from build123d import *

# Parameters (mm, degrees)
SKETCH2_R           = 2.5
BOSS_EXTRUDE1_DEPTH = 3.8
SKETCH3_R           = 2.95
BOSS_EXTRUDE3_DEPTH = 1
SKETCH4_W           = 0.865778577
SKETCH4_H           = 6.939291368
CUT_EXTRUDE1_DEPTH  = 1


with BuildPart() as part:
    # Sketch2 → Boss-Extrude1 (new, symmetric)
    with BuildSketch(Plane(origin=(0, 0, 0), x_dir=(0, 0, -1), z_dir=(1, 0, 0))):
        with Locations(Location((0, 0, 0), (0, 0, 180))):
            Circle(SKETCH2_R)
    extrude(amount=BOSS_EXTRUDE1_DEPTH, both=True)

    # Sketch3 → Boss-Extrude3 (add)
    with BuildSketch(Plane(origin=(3.8, 0, 0), x_dir=(0, 0, -1), z_dir=(1, 0, 0))):
        Circle(SKETCH3_R)
    extrude(amount=BOSS_EXTRUDE3_DEPTH)

    # Sketch4 → Cut-Extrude1 (cut)
    with BuildSketch(Plane.ZY.offset(-3.8)):
        with Locations((-2.932889289, -0.568577956)):
            Rectangle(SKETCH4_W, SKETCH4_H)
    extrude(amount=-CUT_EXTRUDE1_DEPTH, mode=Mode.SUBTRACT)

    # Sketch5 → Cut-Revolve4 (revolve, cut)
    with BuildSketch(Plane(origin=(0, 0, 0), x_dir=(1, 0, 0), z_dir=(0, 1, 0))):
        with BuildLine():
            Line((-3.8, -0.01), (-3.8, -2.5))
            Line((-3.8, -2.5), (-1.31, -2.5))
            ThreePointArc((-1.31, -2.5), (-3.070695885, -1.770695885), (-3.8, -0.01))
        make_face()
    revolve(axis=Axis((-4.317331634, 0, 0), (1, 0, 0)), mode=Mode.SUBTRACT)


solid = part.part
Build history of the part. All positions in model axes, mm. A direction names the side the tool comes from. Round coordinates to 2 decimals unless told otherwise and drop trailing zeros. Write each loop counter-clockwise with the first axis right and the second up, starting at its lowest first coordinate (ties: lowest second). Pieces come first, ordered by that corner, then holes. Notation, with made-up numbers: (50, 8) -> (101, 8) arc R13 cw to (101, 18) -> close; hole circle Ø3 at (44.5, 65). An arc over 180 degrees is marked (long way). Use one line per item in the form item = value.
Q1. Band-saw the part on B-B, the plane y = 2.6. Write the cut outline in (x, z), then the cut area to 3 significant figures.
Conclusion:
outline = (3.8, -1.39) -> (4.8, -1.39) -> (4.8, 1.39) -> (3.8, 1.39) -> close
area = 2.79 mm²
Q2. Drill centre lines: L1, parallel to X at y = -2.35, z = 1.7; L2, parallel to Y at x = -0.5, z = -1.95; L3, parallel to Z at x = 2.5, y = -1.7. Where is each one in solid material? Low to high.
Conclusion:
L1 = 3.8 to 4.8
L2 = -1.56 to 1.56
L3 = -1.83 to 1.83
Q3. Drop flat-ended pins along their axis: P1, Ø3, axis at x = 2.5, z = -1.5, coming from the -Y side; P2, Ø1.5, axis at y = -2, z = 2, coming from the -X side; P3, Ø3, axis at x = -3, z = -1, coming from the +Y side. Give the stop position or say it passes through.
Conclusion:
P1 = -2.85
P2 = -2.7
P3 = 2.46
Q4. Tool access for faces 1 (the cylindrical face through (1.3, -0.1, -2.5)), 2 (the flat face through (4.8, 0, 0)): list every direction of +Z, -Z, +X, -X, +Y, -Y with a clear straight run to the whole face (end or side of a thin tool).
Conclusion:
face_1 = -X
face_2 = +Z, -Z, +X, +Y, -Y
Q5. Band-saw the part on A-A, the plane x = -0.5. Write the cut outline in (y, z), then the cut area to 3 significant figures.
Conclusion:
outline = circle Ø5 at (0, 0)
area = 19.6 mm²
